Read the model definition and answer for the solid it produces. Units are mm, in the model's axes. A direction names the side the tool comes from. Coordinates: 2 decimals unless noted, no trailing zeros. Write each loop counter-clockwise with the first axis right and the second up, starting at its lowest first coordinate (ties: lowest second). Pieces come first, ordered by that corner, then holes. Notation, with made-up numbers: (-8, 74.5) -> (31, 74.5) arc R12 ccw to (31, 94.5) -> close; hole circle Ø4 at (38, 28). An arc over 180 degrees is marked (long way). Answer in a Markdown table with one row per item. Add a question column.
Item 1: Section A-A on x = 15 is taken. Write down the section's boundary in (y, z).
Item 2: Section C-C on x = 115 is taken. Write down the section's boundary in (y, z).
Item 3: Which of the six approach directions +Z, -Z, +X, -X, +Y, -Y give full straight-line access (tool end or side, diameter ignored) to faces 1 (the face through (30, 67, 2)), 2 (the face through (69, 52, 3))?
Item 4: For a pull along X with two mould halves and no side action, classify faces 3 (the face through (69, 52, 0)), 4 (the face through (80.8, 49.5, 1.5)) as +X half, -X half, draft (parallel to the pull), parting line (faces both ways), or undercut.
Item 5: Straight lines are drawn through the part: line 1 (X direction, y = 122, z = 1.95); line 2 (Y direction, x = 15, z = 1.45); line 3 (Y direction, x = 52.5, z = 1.7). For each, find the intervals that lie inside material, in ascending order. Write a range as from..to.
Item 6: Given pin 1 Ø1 at (y, z) = (51, 0.5) entering from +X; pin 2 Ø0.9 at (x, z) = (141, 1.5) entering from +Y; pin 3 Ø1.5 at (y, z) = (-2, 2) entering from +X; pin 4 Ø1.8 at (x, y) = (24, 122) entering from -Z, each flat-ended and moving along its own axis, determine where each tip first touches the part or whether it passes through.
Item 7: Section D-D on z = 1.3 is taken. Count the separate pieces of the cut face and the enclosed holes in it, then the cut area to 3 significant figures.
Item 8: Section B-B on y = 67 is taken. Write down the section's boundary in (x, z).
Autodesk Inventor part; units mm, degrees
ref_plane "YZ Plane" through (0, 0, 0) normal (1, 0, 0) x (0, 1, 0)
ref_plane "XZ Plane" through (0, 0, 0) normal (0, 1, 0) x (-1, 0, 0)
ref_plane "XY Plane" through (0, 0, 0) normal (0, 0, 1) x (1, 0, 0)
sketch "Sketch1" plane through (0, 0, 0) normal (0, 0, 1) x (1, 0, 0)
  line L0 (0, 0) -> (140, 0)
  line L1 (140, 0) -> (140, 134)
  line L2 (140, 134) -> (0, 134)
  line L3 (0, 134) -> (0, 0)
  line L4 (30, 137) -> (45, 137)
  line L5 (45, 137) -> (45, -3)
  line L6 (45, -3) -> (30, -3)
  line L7 (30, -3) -> (30, 137)
  line L8 (100, 137) -> (110, 137)
  line L9 (110, 137) -> (110, -3)
  line L10 (110, -3) -> (100, -3)
  line L11 (100, -3) -> (100, 137)
  line L12 (-3, 124) -> (0, 124)
  line L13 (0, 124) -> (0, 114)
  line L14 (0, 114) -> (-3, 114)
  line L15 (-3, 114) -> (-3, 124)
  line L16 (-3, 20) -> (0, 20)
  line L17 (0, 20) -> (0, 10)
  line L18 (0, 10) -> (-3, 10)
  line L19 (-3, 10) -> (-3, 20)
  line L20 (-3, 72) -> (0, 72)
  line L21 (0, 72) -> (0, 62)
  line L22 (0, 62) -> (-3, 62)
  line L23 (-3, 62) -> (-3, 72)
  line L24 (140, 109) -> (143, 109)
  line L25 (143, 109) -> (143, 99)
  line L26 (143, 99) -> (140, 99)
  line L27 (140, 99) -> (140, 109)
  line L28 (140, 35) -> (143, 35)
  line L29 (143, 35) -> (143, 25)
  line L30 (143, 25) -> (140, 25)
  line L31 (140, 25) -> (140, 35)
  dimension "d0" = 140
  dimension "d1" = 134
  dimension "d2" = 140
  dimension "d3" = 3
  dimension "d4" = 15
  dimension "d5" = 10
  dimension "d6" = 140
  dimension "d7" = 3
  dimension "d8" = 30
  dimension "d9" = 30
  dimension "d10" = 10
  dimension "d11" = 3
  dimension "d13" = 10
  dimension "d14" = 3
  dimension "d16" = 10
  dimension "d17" = 10
  dimension "d74" = 10
  dimension "d75" = 42
  dimension "d76" = 3
  dimension "d77" = 10
  dimension "d78" = 3
  dimension "d79" = 25
  dimension "d80" = 10
  dimension "d81" = 25
  dimension "d82" = 3
extrude "Extrusion1" add sketch "Sketch1" along normal blind 3
sketch "Sketch2" plane through (0, 0, 3) normal (0, 0, 1) x (1, 0, 0)
  line L0 (40, 77) -> (122, 77)
  line L1 (132, 67) -> (132, 67)
  line L2 (122, 57) -> (40, 57)
  line L3 (30, 67) -> (30, 67)
  arc A0 (40, 77) -> (30, 67) centre (40, 67) ccw
  arc A1 (30, 67) -> (40, 57) centre (40, 67) ccw
  arc A2 (122, 57) -> (132, 67) centre (122, 67) ccw
  arc A3 (132, 67) -> (122, 77) centre (122, 67) ccw
  line L4 (140, 114) -> (140, 20)
  line L5 (45, 134) -> (100, 134)
  circle A4 centre (81, 67) radius 17.5
  point P0 (30, 77)
  point P1 (132, 77)
  point P2 (30, 57)
  dimension "d20" = 20
  dimension "d21" = 102
  dimension "d23" = 10
  dimension "d52" = 8
  dimension "d71" = 57
  dimension "d83" = 35
  dimension "d84" = 51
extrude "Extrusion2" cut sketch "Sketch2" against normal through all
sketch "Sketch3" plane through (0, 0, 3) normal (0, 0, 1) x (1, 0, 0)
  line L0 (0, 20) -> (0, 114)
  line L1 (0, 0) -> (0, 10)
  line L2 (30, 0) -> (0, 0)
  line L3 (0, 134) -> (30, 134)
  point P0 (15, 12)
  point P1 (15, 122)
  dimension "d26" = 15
  dimension "d27" = 12
  dimension "d28" = 15
  dimension "d48" = 12
hole "Hole1" at (15, 12, 3) at (15, 122, 3) direction (0, 0, -1) diameter 4 end through all
sketch "Sketch4" plane through (0, 0, 3) normal (0, 0, 1) x (1, 0, 0)
  circle A0 centre (15, 12) radius 2
  circle A1 centre (15, 122) radius 2
  point P0 (24, 122)
  point P1 (6, 122)
  point P2 (24, 12)
  point P3 (6, 12)
  dimension "d37" = 9
  dimension "d38" = 9
  dimension "d39" = 9
  dimension "d40" = 9
  dimension "d49" = 0
  dimension "d50" = 0
hole "Hole2" at (24, 122, 3) at (6, 122, 3) at (24, 12, 3) at (6, 12, 3) direction (0, 0, -1) diameter 3 end through all
sketch "Sketch5" plane through (0, 0, 3) normal (0, 0, 1) x (1, 0, 0)
  point P0 (15, 67)
hole "Hole3" at (15, 67, 3) direction (0, 0, -1) diameter 13 end through all
fillet "圓角1" radius 5 4 edges at (66.6386, 77, 1.5) (95.3614, 77, 1.5) (95.3614, 57, 1.5) (66.6386, 57, 1.5)
sketch "草圖7" plane through (0, 0, 3) normal (0, 0, 1) x (1, 0, 0)
  line L0 (0, 134) -> (9.175, 134)
  line L1 (9.175, 134) -> (9.175, 132.75)
  line L2 (7.925, 131.5) -> (0, 131.5)
  line L3 (0, 131.5) -> (0, 134)
  arc A0 (7.925, 131.5) -> (9.175, 132.75) centre (7.925, 132.75) ccw
  line L4 (0, 0) -> (9.175, 0)
  line L5 (9.175, 0) -> (9.175, 1.25)
  line L6 (7.925, 2.5) -> (0, 2.5)
  line L7 (0, 2.5) -> (0, 0)
  arc A1 (9.175, 1.25) -> (7.925, 2.5) centre (7.925, 1.25) ccw
  point P0 (9.175, 131.5)
  point P1 (9.175, 2.5)
  dimension "d86" = 9.175
  dimension "d88" = 2.5
  dimension "d89" = 1.25
  dimension "d90" = 9.175
  dimension "d91" = 2.5
  dimension "d92" = 1.25
extrude "擠出3" cut sketch "草圖7" against normal through all
equation "\"d93\" = d88"
properties part number "plastic_part_04"
Results below:
| question | item | result |
|---|---|---|
| 1 | outline | (0, 0) -> (10, 0) -> (10, 3) -> (0, 3) -> close; (14, 0) -> (60.5, 0) -> (60.5, 3) -> (14, 3) -> close; (73.5, 0) -> (120, 0) -> (120, 3) -> (73.5, 3) -> close; (124, 0) -> (134, 0) -> (134, 3) -> (124, 3) -> close |
| 2 | outline | (0, 0) -> (57, 0) -> (57, 3) -> (0, 3) -> close; (77, 0) -> (134, 0) -> (134, 3) -> (77, 3) -> close |
| 3 | face 1 | +Z, -Z |
| 3 | face 2 | +Z, +X, -X, +Y, -Y |
| 4 | face 3 | draft |
| 4 | face 4 | undercut |
| 5 | line 1 | x = -3..4.5, 7.5..13, 17..22.5, 25.5..140 |
| 5 | line 2 | y = 0..10, 14..60.5, 73.5..120, 124..134 |
| 5 | line 3 | y = 0..57, 77..134 |
| 6 | pin 1 | stops at x = 140 |
| 6 | pin 2 | stops at y = 109 |
| 6 | pin 3 | stops at x = 110 |
| 6 | pin 4 | passes through |
| 7 | separate pieces | 1 |
| 7 | enclosed holes | 8 |
| 7 | area | 16,600 mm2 |
| 8 | outline | (-3, 0) -> (8.5, 0) -> (8.5, 3) -> (-3, 3) -> close; (21.5, 0) -> (30, 0) -> (30, 3) -> (21.5, 3) -> close; (132, 0) -> (140, 0) -> (140, 3) -> (132, 3) -> close |
